Read the model definition and answer for the solid it produces. Units are mm, in the model's axes. A direction names the side the tool comes from. Coordinates: 2 decimals unless noted, no trailing zeros. Write each loop counter-clockwise with the first axis right and the second up, starting at its lowest first coordinate (ties: lowest second). Pieces come first, ordered by that corner, then holes. Notation, with made-up numbers: (-8, 1.5) -> (34, 1.5) arc R11 ccw to (34, 19.5) -> close; hole circle Ø1 at (-12, 6.5). An arc over 180 degrees is marked (long way). Answer in a Markdown table with one row per item. Add a question column.
Item 1: Section C-C on x = 11 is taken. Write down the section's boundary in (y, z).
Item 2: Section B-B on z = -6 is taken. Write down the section's boundary in (x, y) (3 decimals).
Item 3: For a pull along Z with two mould halves and no side action, classify faces 1 (the face through (-30, -2, -21)), 2 (the face through (0, -2, 0)), 3 (the face through (-23.593, -4.211, -32.705)) as +Z half, -Z half, draft (parallel to the pull), parting line (faces both ways), or undercut.
Item 4: Section A-A on x = -20 is taken. Write down the section's boundary in (y, z) (3 decimals), then the cut area to 3 significant figures.
Item 5: Which of the six approach directions +Z, -Z, +X, -X, +Y, -Y give full straight-line access (tool end or side, diameter ignored) to faces 4 (the face through (15.13, -4.21, -5.79)), 5 (the face through (21.935, -1.676, -4.226))?
Item 6: Section D-D on y = -1.4 is taken. Count the separate pieces of the cut face and the enclosed holes in it, then the cut area to 3 significant figures.
Item 7: Given pin 1 Ø4 at (x, z) = (20, -36) entering from +Y; pin 2 Ø6 at (x, z) = (-20, -36) entering from -Y, each flat-ended and moving along its own axis, determine where each tip first touches the part or whether it passes through.
Item 8: Straight lines are drawn through the part: line 1 (Z direction, x = 11, y = -3.4); line 2 (Z direction, x = 0, y = -1.05); line 3 (X direction, y = -1.3, z = -38). For each, find the intervals that lie inside material, in ascending order. Write a range as from..to.
```python
from build123d import *

# Parameters (mm, degrees)
F0_W           = 11.5
F0_H           = 42
F0_W_2         = 37
F1_DEPTH       = 5
F3_D           = 5.25
F3_DEPTH       = 50
F3_CBORE_D     = 9.75
F3_CBORE_DEPTH = 1.6
F3_TIP         = 1.5772591249
F4_D           = 2.5


with BuildPart() as f1:
    # F0 (on Front) → F1 (new body)
    with BuildSketch(Plane.XZ):
        with Locations((-24.25, -21)):
            Rectangle(F0_W, F0_H)
        with Locations((0, -21)):
            Rectangle(F0_W_2, F0_H)
        with Locations((24.25, -21)):
            Rectangle(F0_W, F0_H)
    extrude(amount=F1_DEPTH)

    # F3
    with Locations(Plane.XZ.offset(5)):
        with Locations((-20, -6), (20, -6), (20, -36), (-20, -36)):
            CounterBoreHole(F3_D / 2, F3_CBORE_D / 2, F3_CBORE_DEPTH, depth=F3_DEPTH)
            with Locations((0, 0, -(F3_DEPTH + F3_TIP / 2))):  # 118° drill point
                Cone(0, F3_D / 2, F3_TIP, mode=Mode.SUBTRACT)

    # F4 (through all)
    with Locations(Plane.XZ.offset(5)):
        with Locations((0, -12.4333016574), (0, -20.4333016574), (-11, -20.4333016574), (11, -20.4333016574)):
            Hole(F4_D / 2)


solid = f1.part
```
Results below:
| question | item | result |
|---|---|---|
| 1 | outline | (-5, -42) -> (0, -42) -> (0, -21.68) -> (-5, -21.68) -> close; (-5, -19.18) -> (0, -19.18) -> (0, 0) -> (-5, 0) -> close |
| 2 | outline | (-30, -5) -> (-24.875, -5) -> (-24.875, -3.4) -> (-22.625, -3.4) -> (-22.625, 0) -> (-30, 0) -> close; (-17.375, -3.4) -> (-15.125, -3.4) -> (-15.125, -5) -> (15.125, -5) -> (15.125, -3.4) -> (17.375, -3.4) -> (17.375, 0) -> (-17.375, 0) -> close; (22.625, -3.4) -> (24.875, -3.4) -> (24.875, -5) -> (30, -5) -> (30, 0) -> (22.625, 0) -> close |
| 3 | face 1 | draft |
| 3 | face 2 | +Z half |
| 3 | face 3 | undercut |
| 4 | outline | (-5, -42) -> (0, -42) -> (0, -38.625) -> (-3.4, -38.625) -> (-3.4, -40.875) -> (-5, -40.875) -> close; (-5, -31.125) -> (-3.4, -31.125) -> (-3.4, -33.375) -> (0, -33.375) -> (0, -8.625) -> (-3.4, -8.625) -> (-3.4, -10.875) -> (-5, -10.875) -> close; (-5, -1.125) -> (-3.4, -1.125) -> (-3.4, -3.375) -> (0, -3.375) -> (0, 0) -> (-5, 0) -> close |
| 4 | area | 143 mm2 |
| 5 | face 4 | -Y |
| 5 | face 5 | +Y, -Y |
| 6 | separate pieces | 1 |
| 6 | enclosed holes | 8 |
| 6 | area | 2,410 mm2 |
| 7 | pin 1 | passes through |
| 7 | pin 2 | stops at y = -3.4 |
| 8 | line 1 | z = -42..-21.68, -19.18..0 |
| 8 | line 2 | z = -42..-21.68, -19.18..-13.68, -11.18..0 |
| 8 | line 3 | x = -30..-21.7, -18.3..18.3, 21.7..30 |
